Could you check a few things on this model? Use its own coordinates, in mm. Face numbers are marked on the shaded views. A direction names the side the tool comes from. Give positions to 0.01 mm unless a question says otherwise; leave off trailing zeros. Write each loop counter-clockwise with the first axis right and the second up, starting at its lowest first coordinate (ties: lowest second). Pieces come first, ordered by that corner, then holes. Notation, with made-up numbers: (24.5, 1) - (59.5, 1) arc R25 ccw to (59.5, 18) - close; hole circle Ø10 at (42.25, -38.5). An arc over 180 degrees is marked (long way). Answer in a Markdown table with one row per item.
from build123d import *

# Parameters (mm, degrees)
F6_W        = 152.1180570126
F6_H        = 74.284017086
F0_DEPTH    = 13.2086668164
F1_DEPTH    = 13.3642852306
F2_W        = 151.2780189514
F2_H        = 29.4950902462
F8_DEPTH    = 20.6191111356
F3_T4_DEPTH = 689.5239445372
F4_DEPTH    = 34.5556028187
F5_R        = 31.0991112757
F9_DEPTH    = 34.5566028187


# Not quite as in the source:
# - a fillet or chamfer that OpenCascade refuses, or shapes differently, is made with other operations: its cross-section is extruded or revolved along the edge and cut away or added


with BuildPart() as f0:
    # F6 (on Top) → F0 (new body)
    with BuildSketch(Plane.XY):
        Rectangle(F6_W, F6_H)
    extrude(amount=F0_DEPTH)

    # F7 (on face) → F1 (join)
    with BuildSketch(Plane.XY.offset(13.2086668164)):
        with BuildLine():
            Line((76.0590285063, 37.142008543), (57.3713417563, 37.142008543))
            ThreePointArc((57.3713417563, 37.142008543), (34.4806875741, 0), (57.3713417563, -37.142008543))
            Line((57.3713417563, -37.142008543), (76.0590285063, -37.142008543))
            Line((76.0590285063, -37.142008543), (76.0590285063, 37.142008543))
        make_face()
        with BuildLine():
            ThreePointArc((57.3713417563, -37.142008543), (97.873650022, -35.396055187), (117.6373694385, 0))
            ThreePointArc((117.6373694385, 0), (97.873650022, 35.396055187), (57.3713417563, 37.142008543))
            Line((57.3713417563, 37.142008543), (76.0590285063, 37.142008543))
            Line((76.0590285063, 37.142008543), (76.0590285063, -37.142008543))
            Line((76.0590285063, -37.142008543), (57.3713417563, -37.142008543))
        make_face()
    extrude(amount=-F1_DEPTH)

    # F2 (on face) → F8 (join)
    with BuildSketch(Plane.XY.offset(13.2086668164)):
        Rectangle(F2_W, F2_H)
    extrude(amount=F8_DEPTH)

    # F3: chamfer of 127 x 22.39352655 on 1 edges, made by hand


with BuildPart() as f3_tool2:
    # F3_s3 → F3_t4 (new body)
    with BuildSketch(Plane.XZ.offset(-344.7619722686)):
        Polygon((-75.6390094757, 11.434251402), (51.3609905243, 33.827777952), (-75.6390094757, 33.827777952), align=None)
    extrude(amount=F3_T4_DEPTH)

    split(bisect_by=Plane.XY.offset(13.2086668164), keep=Keep.TOP)


with BuildPart() as f0_1:
    add(f0.part)

    # F3_t1: cut F3_tool2
    add(f3_tool2.part, mode=Mode.SUBTRACT)

    # F4 (add): a face of the model
    f4_faces = [f0_1.faces().sort_by_distance(p)[0] for p in [
        (76.0590285063, 0, -0.1556184143),
    ]]
    extrude(f4_faces, amount=-F4_DEPTH)

    # F5 (on face) → F9 (cut, through all)
    with BuildSketch(Plane.XY.offset(34.3999844044)):
        with Locations((76.0590285063, 0)):
            Circle(F5_R)
    extrude(amount=-F9_DEPTH, mode=Mode.SUBTRACT)


solid = f0_1.part
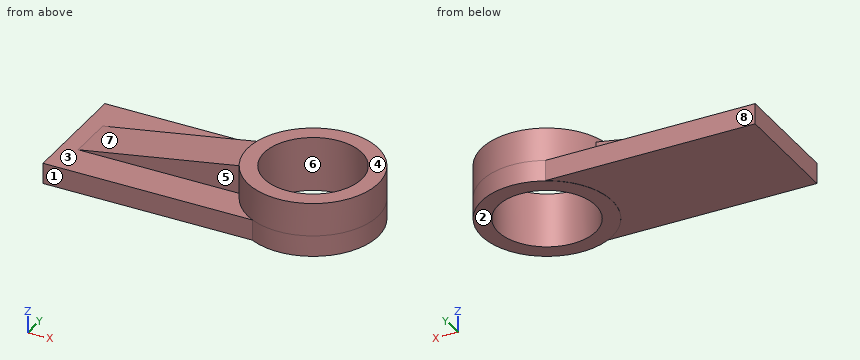
1) If I drill on line 1 (Y direction, x = 77, z = 24); line 2 (Y direction, x = 37, z = 19.5); line 3 (Y direction, x = 50.5, z = 13), over which ranges is the centre line in solid material (lowest first)?
Check values:
| item | result |
|---|---|
| line 1 | y = -41.57 to -31.08, 31.08 to 41.57 |
| line 2 | y = -14.75 to 14.75 |
| line 3 | y = -37.14 to -17.72, 17.72 to 37.14 |
2) Will these pins go through, and if not, where does the flat tip stop? P1, Ø3, axis at x = 3, z = 22.5, coming from the +Y side; P2, Ø3, axis at y = 22.5, z = 21, coming from the +X side; P3, Ø10.5, axis at x = -26.5, z = 4.5, coming from the +Y side.
Check values:
| item | result |
|---|---|
| P1 | stops at y = 14.75 |
| P2 | stops at x = 111.94 |
| P3 | stops at y = 37.14 |
3) We'd pull the mould along X, two halves only. Please class the marked faces 6, 7 and 8: +X half, -X half, draft (parallel to the pull), parting line (faces both ways), or undercut.
Check values:
| item | result |
|---|---|
| face 6 | undercut |
| face 7 | -X half |
| face 8 | draft |
4) Imagine slicing it at B-B (x = 51.5). List the corners of the cut face in (y, z) for me.
Check values:
| item | result |
|---|---|
| outline | (-37.14, 0) - (-33.55, 0) - (-33.55, -0.16) - (-19.08, -0.16) - (-19.08, 34.4) - (-33.55, 34.4) - (-33.55, 13.21) - (-37.14, 13.21) - close; (19.08, -0.16) - (33.55, -0.16) - (33.55, 0) - (37.14, 0) - (37.14, 13.21) - (33.55, 13.21) - (33.55, 34.4) - (19.08, 34.4) - close |
5) Imagine slicing it at C-C (z = 4.5). List the corners of the cut face in (x, y) for me.
Check values:
| item | result |
|---|---|
| outline | (-76.06, -37.14) - (57.37, -37.14) arc R41.58 ccw (long way) to (57.37, 37.14) - (-76.06, 37.14) - close; hole circle Ø62.2 at (76.06, 0) |
6) Imagine slicing it at A-A (y = -11.5). List the corners of the cut face in (x, z) for me.
Check values:
| item | result |
|---|---|
| outline | (-76.06, 0) - (36.1, 0) - (36.1, -0.16) - (47.16, -0.16) - (47.16, 34.4) - (36.1, 34.4) - (36.1, 31.14) - (-65.58, 13.21) - (-76.06, 13.21) - close; (104.95, -0.16) - (116.02, -0.16) - (116.02, 34.4) - (104.95, 34.4) - close |
7) Imagine slicing it at D-D (y = 33). List the corners of the cut face in (x, z) for me, then the cut area to 3 significant figures.
Check values:
| item | result |
|---|---|
| outline | (-76.06, 0) - (50.77, 0) - (50.77, -0.16) - (101.35, -0.16) - (101.35, 34.4) - (50.77, 34.4) - (50.77, 13.21) - (-76.06, 13.21) - close |
| area | 3,420 mm2 |
8) On a 3-axis mill with a long thin cutter (end or side, diameter ignored), from which of +Z, -Z, +X, -X, +Y, -Y can I reach the whole of each face in a straight line? I mean the marked faces 1, 2, 3, 4 and 5. Say none if no direction works.
Check values:
| item | result |
|---|---|
| face 1 | +Z, -Z, -X, -Y |
| face 2 | -Z, +X, -X, +Y, -Y |
| face 3 | +Z, -X |
| face 4 | +Z, +X, -X, +Y, -Y |
| face 5 | +Z, -X, -Y |
